```python
from build123d import *

# Parameters (mm, degrees)
F1_DEPTH = 12.7
F3_DEPTH = 3.81
F4_R     = 3.81
F5_DEPTH = 6.35


with BuildPart() as f1:
    # F0 (on Top) → F1 (new body)
    with BuildSketch(Plane.XY):
        with BuildLine():
            ThreePointArc((5.030861, -0.704865), (5.0677, -0.353288), (5.08, 0))
            ThreePointArc((5.08, 0), (4.212113, 2.839806), (1.905, 4.709286))
            ThreePointArc((1.905, 4.709286), (0, 5.08), (-1.905, 4.709286))
            ThreePointArc((-1.905, 4.709286), (-4.399409, 2.54), (-5.030861, -0.704865))
            ThreePointArc((-5.030861, -0.704865), (-4.399409, -2.54), (-3.125861, -4.004421))
            ThreePointArc((-3.125861, -4.004421), (0, -5.08), (3.125861, -4.004421))
            ThreePointArc((3.125861, -4.004421), (4.399409, -2.54), (5.030861, -0.704865))
        make_face()
    extrude(amount=F1_DEPTH)

    # F2 (on Top) → F3 (join)
    with BuildSketch(Plane.XY):
        with BuildLine():
            Line((10.530123, -3.879865), (5.030861, -0.704865))
            ThreePointArc((5.030861, -0.704865), (4.399409, -2.54), (3.125861, -4.004421))
            Line((3.125861, -4.004421), (8.625123, -7.179421))
            Line((8.625123, -7.179421), (10.530123, -3.879865))
        make_face()
        with BuildLine():
            ThreePointArc((-1.905, 4.709286), (0, 5.08), (1.905, 4.709286))
            Line((1.905, 4.709286), (1.905, 11.059286))
            Line((1.905, 11.059286), (-1.905, 11.059286))
            Line((-1.905, 11.059286), (-1.905, 4.709286))
        make_face()
        with BuildLine():
            ThreePointArc((-3.125861, -4.004421), (-4.399409, -2.54), (-5.030861, -0.704865))
            Line((-5.030861, -0.704865), (-10.530123, -3.879865))
            Line((-10.530123, -3.879865), (-8.625123, -7.179421))
            Line((-8.625123, -7.179421), (-3.125861, -4.004421))
        make_face()
    extrude(amount=F3_DEPTH)

    # F4 (on face) → F5 (cut)
    with BuildSketch(Plane.XY.offset(12.7)):
        Circle(F4_R)
    extrude(amount=-F5_DEPTH, mode=Mode.SUBTRACT)


solid = f1.part
```
Can you work these out from the model? Positions are in its coordinate system, mm. A direction names the side the tool comes from. Give positions to 0.01 mm unless a question says otherwise; leave off trailing zeros. Write each loop counter-clockwise with the first axis right and the second up, starting at its lowest first coordinate (ties: lowest second). Pieces come first, ordered by that corner, then holes. Notation, with made-up numbers: (71, 84.25) - (109, 84.25) arc R27 ccw to (109, 105.25) - close; hole circle Ø7 at (-1, -2.5). An arc over 180 degrees is marked (long way). Write item = value, one per line. Start each with the question number.
1. For pin 1 (4 mm diameter, centred on x = -1.5, z = 8.5, fed in from +Y); pin 2 (7 mm diameter, centred on x = 8, y = -5, fed in from +Z); pin 3 (1.9 mm diameter, centred on y = 8, z = 2.5, fed in from +X) (3 decimals), each with a flat end and sliding along its axis, tell me the tip position at first contact or that it passes through.
2. Imagine slicing it at C-C (z = 2.75). Please give me the cut outline in (x, y) (3 decimals), and give its area (3 significant figures).
3. On a 3-axis mill with a long thin cutter (end or side, diameter ignored), from which of +Z, -Z, +X, -X, +Y, -Y can I reach the whole of each face in a straight line? I mean faces 5 (the face through (-0.83, -3.72, 9.57)), 6 (the face through (1.905, 8, 2)), 7 (the face through (-5.91, -5.61, 1.88)). Say none if no direction works.
4. Imagine slicing it at B-B (x = 0). Please give me the cut outline in (y, z), and give its area (3 significant figures).
5. Thinking about a two-plate mould opening in Y: for faces 1 (the face through (0, 0, 6.35)), 2 (the face through (5.84, -5.57, 1.88)), 3 (the face through (-7, -4, 3.81)), 4 (the face through (-7.74, -2.27, 1.88)), which applies, released by +Y, released by -Y, zero draft, split by the parting line, or undercut?
6. Please list where these lines run through material, in increasing order: line 1 (Y direction, x = 0, z = 9.75); line 2 (X direction, y = 6, z = 0.5) (3 decimals); line 3 (X direction, y = -1.5, z = 6.75).
7. Imagine slicing it at A-A (z = 9). Please give me the cut outline in (x, y) (3 decimals), and give its area (3 significant figures).
8. Imagine slicing it at D-D (y = 3.5). Please give me the cut outline in (x, z).
Worked answers:
q1.pin_1 = 5.08
q1.pin_2 = 3.81
q1.pin_3 = 1.905
q2.outline = (-10.53, -3.88) - (-8.625, -7.179) - (-3.126, -4.004) arc R5.08 ccw to (3.126, -4.004) - (8.625, -7.179) - (10.53, -3.88) - (5.031, -0.705) arc R5.08 ccw to (5.08, 0) arc R5.08 ccw to (1.905, 4.709) - (1.905, 11.059) - (-1.905, 11.059) - (-1.905, 4.709) arc R5.08 ccw to (-5.031, -0.705) - close
q2.area = 151 mm2
q3.face_5 = +Z
q3.face_6 = +Z, -Z, +X, +Y
q3.face_7 = +Z, -Z, -Y
q4.outline = (-5.08, 0) - (11.06, 0) - (11.06, 3.81) - (5.08, 3.81) - (5.08, 12.7) - (3.81, 12.7) - (3.81, 6.35) - (-3.81, 6.35) - (-3.81, 12.7) - (-5.08, 12.7) - close
q4.area = 103 mm2
q5.face_1 = undercut
q5.face_2 = released by -Y
q5.face_3 = zero draft
q5.face_4 = released by +Y
q6.line_1 = -5.08 to -3.81, 3.81 to 5.08
q6.line_2 = -1.905 to 1.905
q6.line_3 = -4.85 to -3.5, 3.5 to 4.85
q7.outline = (-5.031, -0.705) arc R5.08 ccw to (-3.126, -4.004) arc R5.08 ccw to (3.126, -4.004) arc R5.08 ccw to (5.031, -0.705) arc R5.08 ccw to (5.08, 0) arc R5.08 ccw to (1.905, 4.709) arc R5.08 ccw to start; hole circle Ø7.62 at (0, 0)
q7.area = 35.5 mm2
q8.outline = (-3.68, 0) - (3.68, 0) - (3.68, 12.7) - (1.51, 12.7) - (1.51, 6.35) - (-1.51, 6.35) - (-1.51, 12.7) - (-3.68, 12.7) - close
